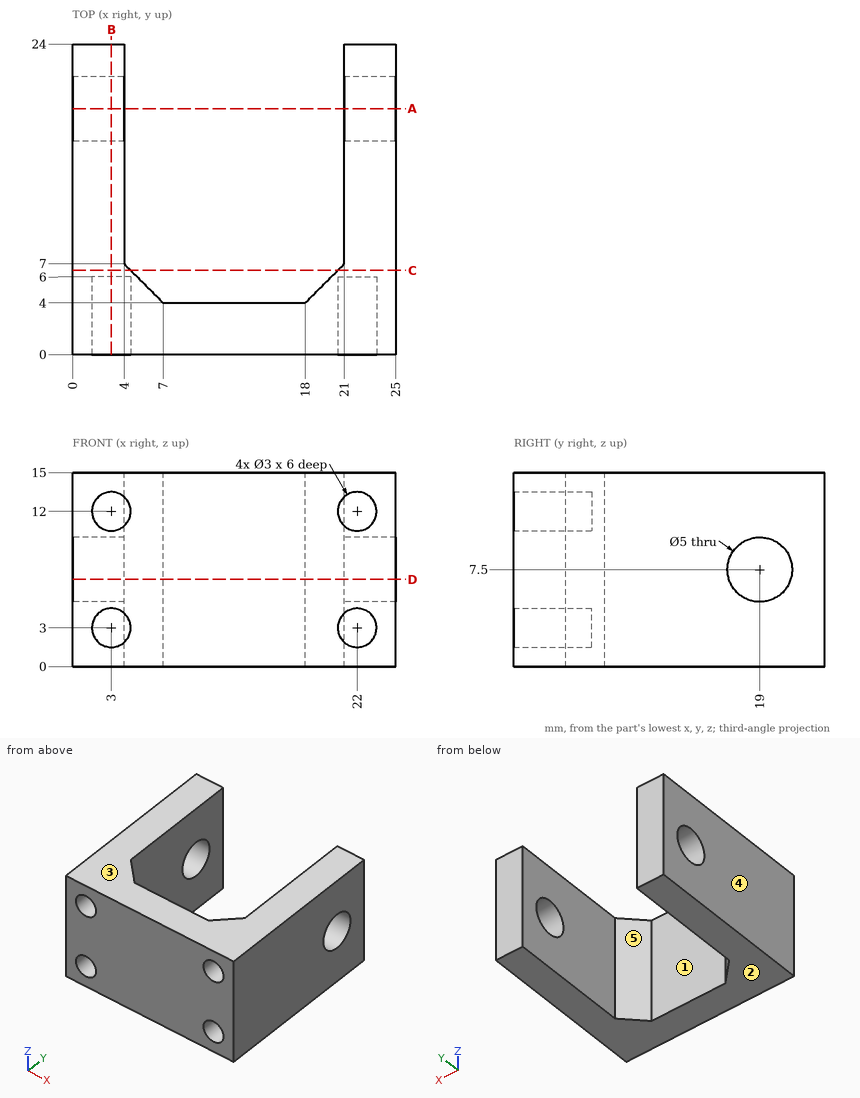
Check sheet for the drawn part. Datum: minimum x, y, z corner. Units: mm. A direction names the side the tool comes from. Round coordinates to 2 decimals unless told otherwise and drop trailing zeros. Write each loop counter-clockwise with the first axis right and the second up, starting at its lowest first coordinate (ties: lowest second). Pieces come first, ordered by that corner, then holes. Notation, with made-up numbers: (31, -39) -> (43, -39) arc R24 cw to (43, -29) -> close; hole circle Ø4 at (78, -23). An arc over 180 degrees is marked (long way). Write each question's results on one line, items separated by ' | '.
Q1. Access from +Z, -Z, +X, -X, +Y, -Y to the whole of each face (thin tool, end or side, straight path). Record for the marked faces 1 and 2.
Derived:
face 1: +Z, -Z, +Y | face 2: -Z, +X, -X, +Y, -Y
Q2. Draft check along X on the marked faces 3, 4 and 5. Enter one of: released by +X, released by -X, zero draft, split by the parting line, or undercut.
Derived:
face 3: zero draft | face 4: released by -X | face 5: undercut
Q3. Thickness scan on probe 1 along X at (y, z) = (2.7, 12); probe 2 along X at (y, z) = (8, 10.25); probe 3 along Z at (x, y) = (2.8, 19). Record the ranges inside material, lowest first.
Derived:
probe 1: x = 0 to 1.5, 4.5 to 20.5, 23.5 to 25 | probe 2: x = 0 to 4, 21 to 25 | probe 3: z = 0 to 5, 10 to 15
Q4. Sectioned sample at A-A, the plane y = 19. Record the boundary of the cut face in (x, z), and give its area (3 significant figures).
Derived:
outline: (0, 0) -> (4, 0) -> (4, 5) -> (0, 5) -> close; (0, 10) -> (4, 10) -> (4, 15) -> (0, 15) -> close; (21, 0) -> (25, 0) -> (25, 5) -> (21, 5) -> close; (21, 10) -> (25, 10) -> (25, 15) -> (21, 15) -> close | area: 80.0 mm²
Q5. Sectioned sample at D-D, the plane z = 6.75. Record the boundary of the cut face in (x, y), and give its area (3 significant figures).
Derived:
outline: (0, 0) -> (25, 0) -> (25, 16.62) -> (21, 16.62) -> (21, 7) -> (18, 4) -> (7, 4) -> (4, 7) -> (4, 16.62) -> (0, 16.62) -> close; (0, 21.38) -> (4, 21.38) -> (4, 24) -> (0, 24) -> close; (21, 21.38) -> (25, 21.38) -> (25, 24) -> (21, 24) -> close | area: 231 mm²
Q6. Go/stop test with flat-tipped pins: pin 1 Ø2.5 at (x, z) = (22, 3) entering from -Y; pin 2 Ø10 at (x, y) = (11, 17.5) entering from -Z; pin 3 Ø3.5 at (x, z) = (12.5, 10) entering from +Y. Record where each tip stops, or that it passes through.
Derived:
pin 1: stops at y = 6 | pin 2: passes through | pin 3: stops at y = 4
Q7. Sectioned sample at B-B, the plane x = 3. Record the boundary of the cut face in (y, z), and give its area (3 significant figures).
Derived:
outline: (0, 0) -> (24, 0) -> (24, 15) -> (0, 15) -> (0, 13.5) -> (6, 13.5) -> (6, 10.5) -> (0, 10.5) -> (0, 4.5) -> (6, 4.5) -> (6, 1.5) -> (0, 1.5) -> close; hole circle Ø5 at (19, 7.5) | area: 304 mm²
Q8. Sectioned sample at C-C, the plane y = 6.5. Record the boundary of the cut face in (x, z), and give its area (3 significant figures).
Derived:
outline: (0, 0) -> (4.5, 0) -> (4.5, 15) -> (0, 15) -> close; (20.5, 0) -> (25, 0) -> (25, 15) -> (20.5, 15) -> close | area: 135 mm²
